Autodesk Inventor part; units mm, degrees
ref_plane "YZ Plane" through (0, 0, 0) normal (1, 0, 0) x (0, 1, 0)
ref_plane "XZ Plane" through (0, 0, 0) normal (0, 1, 0) x (-1, 0, 0)
ref_plane "XY Plane" through (0, 0, 0) normal (0, 0, 1) x (1, 0, 0)
sketch "Sketch1" plane through (0, 0, 0) normal (0, 0, 1) x (1, 0, 0)
  line L0 (0, 0) -> (0, 14.844)
  line L1 (-5.08, 16.2052) -> (-5.08, 0)
  line L2 (-5.08, 0) -> (0, 0)
  line L3 (-5.08, 16.2052) -> (14.2875, 49.7507)
  line L4 (14.2875, 49.7507) -> (-9.646, 91.2048)
  line L5 (-9.646, 91.2048) -> (-5.2466, 93.7448)
  line L6 (-5.2466, 93.7448) -> (20.1534, 49.7507)
  line L7 (20.1534, 49.7507) -> (0, 14.844)
  line L8 (-5.2466, 93.7448) -> (-0.1666, 74.786)
  dimension "d0" = 16.2052
  dimension "d1" = 5.08
  dimension "d6" = 5.08
  dimension "d7" = 5.08
  dimension "d8" = 30
  dimension "d10" = 120
  dimension "d11" = 50.8
  dimension "d12" = 38.735
  dimension "d13" = 15
extrude "Extrusion1" add sketch "Sketch1" along normal blind 20.32 contours L2 L1 L3 L4 L8 L6 L7 L0
fillet "Fillet1" radius 1.5875 1 edges at (-5.2466, 93.7448, 10.16)
ref_plane "Work Plane1" through (-10.16, 0, 0) normal (-1, 0, 0) x (0, 0, 1)
sketch "Sketch2" plane through (-10.16, 0, 0) normal (-1, 0, 0) x (0, 0, 1)
  line L0 (0, 0) -> (20.32, 0)
  line L1 (3.937, 0) -> (16.383, 0)
  line L2 (16.383, 0) -> (16.383, 24.9936)
  line L3 (16.383, 24.9936) -> (3.937, 24.9936)
  line L4 (3.937, 24.9936) -> (3.937, 0)
  point P0 (10.16, 0)
  point P1 (16.383, 0)
  dimension "d16" = 12.446
  dimension "d17" = 24.9936
  dimension "d18" = 6.223
extrude "Extrusion2" add sketch "Sketch2" against normal up to next
sketch "Sketch3" plane through (0, 0, 0) normal (1, 0, 0) x (0, 0, -1)
  circle A0 centre (-10.16, 7.422) radius 1.778
  line L0 (0, 0) -> (0, 14.844)
  line L1 (0, 0) -> (-20.32, 0)
  point P0 (0, 7.422)
  point P1 (-10.16, 0)
  dimension "d23" = 3.556
extrude "Extrusion3" cut sketch "Sketch3" against normal blind 15.875
sketch "Sketch4" plane through (0, 0, 0) normal (1, 0, 0) x (0, 0, -1)
  circle A0 centre (-10.16, 7.422) radius 1.778
  circle A1 centre (-10.16, 7.422) radius 3.81
  point P0 (0, 0)
  dimension "d24" = 7.62
extrude "Extrusion4" cut sketch "Sketch4" against normal blind 4.0132 contours A0 | A1
properties part number "KNUCKLE 1"
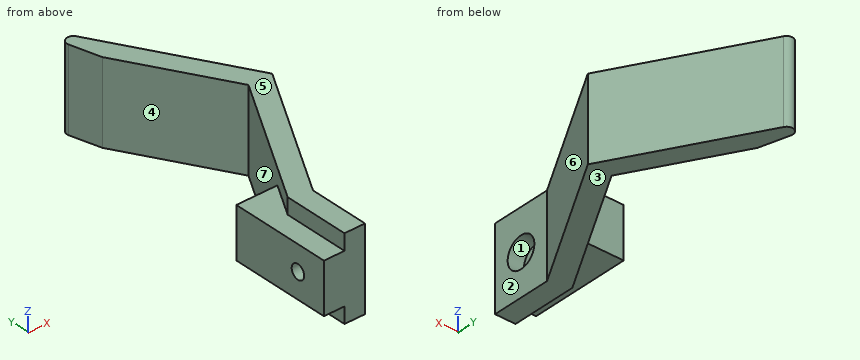
The listing builds one solid part. Answer for the finished solid, in the listing's coordinates (mm). Face numbers are marked on the shaded views. A direction names the side the tool comes from. Coordinates: 2 decimals unless noted, no trailing zeros. Write each loop counter-clockwise with the first axis right and the second up, starting at its lowest first coordinate (ties: lowest second). Pieces come first, ordered by that corner, then holes. Notation, with made-up numbers: (43.5, -17.75) - (64.5, -17.75) arc R36 ccw to (64.5, 16.25) - close; hole circle Ø7 at (17, 83.5). An arc over 180 degrees is marked (long way). Return JSON: item names as keys, results as strings. Group by question number.
1. Given pin 1 (3 mm diameter, centred on x = -2.5, y = 11, fed in from -Z); pin 2 (4.5 mm diameter, centred on y = 8, z = 1, fed in from -X); pin 3 (1.5 mm diameter, centred on x = 1.5, z = 10.5, fed in from -Y); pin 4 (12 mm diameter, centred on y = 9.5, z = 12, fed in from +X), each flat-ended and moving along its own axis, determine where each tip first touches the part or whether it passes through.
2. A cutting plane is placed at A-A, the plane z = 10.16. Determine the outline of the cut face in (x, y) (1 decimal), plus the area to 3 significant figures.
3. Which of the six approach directions +Z, -Z, +X, -X, +Y, -Y give full straight-line access (tool end or side, diameter ignored) to the marked faces 1, 2, 3 and 4?
4. A cutting plane is placed at C-C, the plane x = 2. Determine the outline of the cut face in (y, z).
5. A cutting plane is placed at B-B, the plane y = 13. Determine the outline of the cut face in (x, z).
6. A cutting plane is placed at D-D, the plane z = 3. Determine the outline of the cut face in (x, y) (1 decimal), plus the area to 3 significant figures.
7. Determine the mould class of the marked faces 5, 6 and 7 for opening direction Y: released by +Y, released by -Y, zero draft, split by the parting line, or undercut.
8. Straight lines are drawn through the part: L1, parallel to Y at x = -2.3, z = 10.16; L2, parallel to Y at x = -5.25, z = 10.16; L3, parallel to X at y = 12, z = 10.5. For each, find the intervals that lie inside material, in ascending order.
Ans:
{
 "1": {"pin 1": "z = 0", "pin 2": "x = -5.08", "pin 3": "y = 16.14", "pin 4": "x = 0.38"},
 "2": {"outline": "(-10.2, 0) - (0, 0) - (0, 3.6) - (-4, 3.6) - (-4, 5.6) - (-10.2, 5.6) - close; (-10.2, 9.2) - (-4, 9.2) - (-4, 11.2) - (0, 11.2) - (0, 14.8) - (20.2, 49.8) - (0.8, 83.3) arc R1.6 ccw to (-2.1, 82.1) - (-0.2, 74.8) - (14.3, 49.8) - (0, 25) - (-10.2, 25) - close", "area": "563 mm²"},
 "3": {"face 1": "+X", "face 2": "+Z, -Z, +X, -Y", "face 3": "-Z, +X, -X, +Y, -Y", "face 4": "+Z, -Z, -X"},
 "4": {"outline": "(18.31, 0) - (28.47, 0) - (28.47, 20.32) - (18.31, 20.32) - close; (71.03, 0) - (81.19, 0) - (81.19, 20.32) - (71.03, 20.32) - close"},
 "5": {"outline": "(-10.16, 3.94) - (-5.08, 3.94) - (-5.08, 0) - (0, 0) - (0, 20.32) - (-5.08, 20.32) - (-5.08, 16.38) - (-10.16, 16.38) - close"},
 "6": {"outline": "(-5.1, 0) - (0, 0) - (0, 14.8) - (20.2, 49.8) - (0.8, 83.3) arc R1.6 ccw to (-2.1, 82.1) - (-0.2, 74.8) - (14.3, 49.8) - (-5.1, 16.2) - close", "area": "467 mm²"},
 "7": {"face 5": "zero draft", "face 6": "released by -Y", "face 7": "undercut"},
 "8": {"L1": "0 to 3.61, 11.23 to 24.99", "L2": "0 to 5.64, 9.2 to 24.99", "L3": "-10.16 to 0"}
}
